Here's how the part is built. I have some questions about the finished solid (model axes, mm). A direction names the side the tool comes from. Coordinates: 2 decimals unless noted, no trailing zeros. Loops run counter-clockwise (first coordinate to the right, second up) from the corner with the lowest first, then second, coordinate; pieces in that order, holes last. Notation, with made-up numbers: (16, 25.25) - (51, 25.25) arc R30 ccw to (51, 60.25) - close; hole circle Ø6 at (77.5, -31). An arc over 180 degrees is marked (long way). Use a Markdown table: item, result.
Autodesk Inventor part; units mm, degrees
ref_plane "YZ Plane" through (0, 0, 0) normal (1, 0, 0) x (0, 1, 0)
ref_plane "XZ Plane" through (0, 0, 0) normal (0, 1, 0) x (-1, 0, 0)
ref_plane "XY Plane" through (0, 0, 0) normal (0, 0, 1) x (1, 0, 0)
sketch "Sketch3" plane through (0, 0, 0) normal (0, 0, 1) x (1, 0, 0)
  line L0 (0, 0) -> (-10, 0)
  line L1 (-10, 0) -> (-10, 6)
  line L2 (-10, 6) -> (-10.25, 6)
  line L3 (-10.25, 6) -> (-10.25, 8)
  line L4 (-10.25, 8) -> (-12.5, 8)
  line L5 (-12.5, 8) -> (-12.5, 10)
  line L6 (-12.5, 10) -> (-10.5, 10)
  line L7 (-10.5, 10) -> (-10.5, 15)
  line L8 (-10.5, 15) -> (-9.2, 15)
  line L9 (-9.2, 15) -> (-9.2, 17.6)
  line L10 (-9.2, 17.6) -> (-10.5, 17.6)
  line L11 (-10.5, 17.6) -> (-10.5, 22.6)
  line L12 (-10.5, 22.6) -> (0, 22.6)
  line L13 (0, 22.6) -> (0, 0)
  line L14 (0, 22.6) -> (-8, 22.6)
  line L15 (-8, 22.6) -> (-8, 0)
  dimension "d23" = 10
  dimension "d24" = 6
  dimension "d25" = 0.25
  dimension "d26" = 2
  dimension "d27" = 2.25
  dimension "d28" = 2
  dimension "d29" = 2
  dimension "d30" = 5
  dimension "d31" = 1.3
  dimension "d32" = 2.6
  dimension "d33" = 5
  dimension "d34" = 8
revolve "Revolution2" add sketch "Sketch3" angle 360 about axis through (0, 22.6, 0) along (0, -1, 0) contours L0 L1 L2 L3 L4 L5 L6 L7 L8 L9 L10 L11 L12 L15
thread "Thread3"
properties part number "Conector Tapa-Corrugado V2" material "Polypropylene"
Q1. Will these pins go through, and if not, where does the flat tip stop? P1, Ø2, axis at x = -0.5, z = -6, coming from the +Y side; P2, Ø2, axis at y = 15, z = 4.5, coming from the +X side; P3, Ø1, axis at y = 3.5, z = -4.5, coming from the -X side; P4, Ø1, axis at x = -3, y = 8, coming from the +Z side.
Check values:
| item | result |
|---|---|
| P1 | through |
| P2 | x = 9.9 |
| P3 | x = -9.17 |
| P4 | z = 12.25 |
Q2. I want a section at A-A, the plane x = 0. Write out the boundary of the cut face in (y, z), then the cut area to 3 significant figures.
Check values:
| item | result |
|---|---|
| outline | (0, -10) - (6, -10) - (6, -10.25) - (8, -10.25) - (8, -12.5) - (10, -12.5) - (10, -10.5) - (15, -10.5) - (15, -9.2) - (17.6, -9.2) - (17.6, -10.5) - (22.6, -10.5) - (22.6, -8) - (0, -8) - close; (0, 8) - (22.6, 8) - (22.6, 10.5) - (17.6, 10.5) - (17.6, 9.2) - (15, 9.2) - (15, 10.5) - (10, 10.5) - (10, 12.5) - (8, 12.5) - (8, 10.25) - (6, 10.25) - (6, 10) - (0, 10) - close |
| area | 107 mm^2 |
Q3. I want a section at C-C, the plane y = 13.5. Write out the boundary of the cut face in (x, z).
Check values:
| item | result |
|---|---|
| outline | circle Ø21 at (0, 0); hole circle Ø16 at (0, 0) |
Q4. Which directions (+Z, -Z, +X, -X, +Y, -Y) give clear straight access to the entire face, cutting with the end or side of a thin tool? Please do faces 4 (the face through (-6.2, 17.6, 7)), 5 (the face through (-10, 20.1, 3.2)), 6 (the face through (-11.923, 9.014, 3.755)), 7 (the face through (1.91, 8, -10.24)).
Check values:
| item | result |
|---|---|
| face 4 | none |
| face 5 | +Y |
| face 6 | +Y, -Y |
| face 7 | -Y |
Q5. Please list where these lines run through material, in increasing order: L1, parallel to X at y = 11.5, z = 0; L2, parallel to Z at x = 0, y = 6.25; L3, parallel to X at y = 17.5, z = 0. Write a range as from..to.
Check values:
| item | result |
|---|---|
| L1 | -10.5..-8, 8..10.5 |
| L2 | -10.25..-8, 8..10.25 |
| L3 | -9.2..-8, 8..9.2 |
Q6. I want a section at B-B, the plane z = 0. Write out the boundary of the cut face in (x, y).
Check values:
| item | result |
|---|---|
| outline | (-12.5, 8) - (-10.25, 8) - (-10.25, 6) - (-10, 6) - (-10, 0) - (-8, 0) - (-8, 22.6) - (-10.5, 22.6) - (-10.5, 17.6) - (-9.2, 17.6) - (-9.2, 15) - (-10.5, 15) - (-10.5, 10) - (-12.5, 10) - close; (8, 0) - (10, 0) - (10, 6) - (10.25, 6) - (10.25, 8) - (12.5, 8) - (12.5, 10) - (10.5, 10) - (10.5, 15) - (9.2, 15) - (9.2, 17.6) - (10.5, 17.6) - (10.5, 22.6) - (8, 22.6) - close |
Q7. If we mould it in two halves opening along Y, with no side actions, what happens to faces 1 (the face through (2, 22.6, 8)), 2 (the face through (2.17, 3.04, -9.76)), 3 (the face through (7.3, 16.3, -5.6))? For each: pulls with the +Y half, pulls with the -Y half, needs draft (parallel to the pull), parting line crosses it, or undercut.
Check values:
| item | result |
|---|---|
| face 1 | pulls with the +Y half |
| face 2 | needs draft |
| face 3 | undercut |
